The listing builds one solid part. Answer for the finished solid, in the listing's coordinates (mm). Face numbers are marked on the shaded views. A direction names the side the tool comes from. Round coordinates to 2 decimals unless told otherwise and drop trailing zeros. Order: outer loops, then holes, each group sorted by start corner. A loop starts at its lowest first (then second) coordinate and runs counter-clockwise, first axis right, second up. Notation, with made-up numbers: (27, 66.25) - (80, 66.25) arc R13 ccw to (80, 81.25) - close; hole circle Ø5 at (25, -21.75). An arc over 180 degrees is marked (long way). Use CSV: the item, a comma, the result in double quotes. Start each with the question number.
Item 1: Find section B-B, the plane x = 32.5. Give the vertices of the cut face in (y, z).
Item 2: For the marked faces 1 and 2, determine the directions among +Z, -Z, +X, -X, +Y, -Y from which every point of the face is accessible in a straight line to the end or side of a thin tool.
Item 3: Straight lines are drawn through the part: line 1 along Z through (x, y) = (4, 6); line 2 along X through (y, z) = (39, 47.5); line 3 along Y through (x, z) = (4, 23). For each, find the intervals that lie inside material, in ascending order. Write a range as [from, to].
Item 4: Find section D-D, the plane z = -72. Give the vertices of the cut face in (x, y).
Item 5: Find section A-A, the plane y = 20. Give the vertices of the cut face in (x, z), plus the area to 3 significant figures.
Item 6: Flat-ended cylindrical pins translate along their axes: P1, Ø6, axis at x = 10, y = 13.5, coming from the -Z side; P2, Ø10, axis at y = 57.5, z = 31, coming from the +X side; P3, Ø5, axis at x = 3.5, z = 37.5, coming from the +Y side; P4, Ø1.4, axis at x = 2.5, z = -27.5, coming from the -Y side. Find the tip coordinate at first contact, or state that the pin passes through.
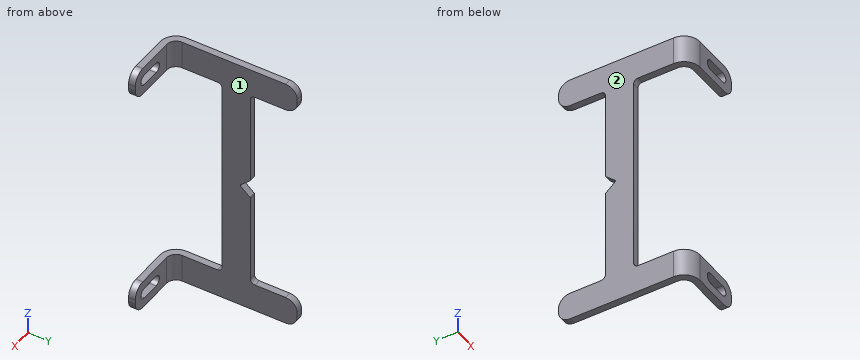
```python
from build123d import *

# Parameters (mm, degrees)
BASE_FLANGE1_DEPTH = 88.9
EXTRUDE2_REACH     = 132.358
EXTRUDE3_REACH     = 133.902
EXTRUDE4_DEPTH     = 134.35
FILLET1_R          = 7.9375
CUT_EXTRUDE1_REACH = 133.902
FILLET2_R          = 0.79375


# Sheet-metal steps are written as plain solids
with BuildPart() as part:
    # Sketch1 → Base-Flange1 (new, symmetric)
    with BuildSketch(Plane.XY):
        with BuildLine():
            Line((0, 88.9), (0, 10.90422))
            ThreePointArc((0, 10.90422), (3.193772094, 3.193772094), (10.90422, 0))
            Line((10.90422, 0), (44.45, 0))
            Line((44.45, 0), (44.45, 4.55422))
            Line((44.45, 4.55422), (10.90422, 4.55422))
            ThreePointArc((10.90422, 4.55422), (6.414091939, 6.414091939), (4.55422, 10.90422))
            Line((4.55422, 10.90422), (4.55422, 88.9))
            Line((4.55422, 88.9), (0, 88.9))
        make_face()
    extrude(amount=BASE_FLANGE1_DEPTH, both=True)

    # Sketch3 → Extrude2 (cut, up to next)
    with BuildSketch(Plane(origin=(0, 4.55422, 0), x_dir=(1, 0, 0), z_dir=(0, 1, 0)), mode=Mode.PRIVATE) as extrude2_sk1:
        with BuildLine():
            Line((34.925, -82.946875), (22.225, -82.946875))
            ThreePointArc((22.225, -82.946875), (18.653125, -79.375), (22.225, -75.803125))
            Line((22.225, -75.803125), (34.925, -75.803125))
            ThreePointArc((34.925, -75.803125), (38.496875, -79.375), (34.925, -82.946875))
        make_face()
    extrude2_tool1 = extrude(extrude2_sk1.sketch, amount=-EXTRUDE2_REACH, mode=Mode.PRIVATE) & part.part
    # Sketch3 → Extrude2 (cut, up to next)
    with BuildSketch(Plane(origin=(0, 4.55422, 0), x_dir=(1, 0, 0), z_dir=(0, 1, 0)), mode=Mode.PRIVATE) as extrude2_sk2:
        with BuildLine():
            Line((34.925, 75.803125), (22.225, 75.803125))
            ThreePointArc((22.225, 75.803125), (18.653125, 79.375), (22.225, 82.946875))
            Line((22.225, 82.946875), (34.925, 82.946875))
            ThreePointArc((34.925, 82.946875), (38.496875, 79.375), (34.925, 75.803125))
        make_face()
    extrude2_tool2 = extrude(extrude2_sk2.sketch, amount=-EXTRUDE2_REACH, mode=Mode.PRIVATE) & part.part
    add(extrude2_tool1.solids().sort_by_distance((28.575, 4.55422, 79.375))[0], mode=Mode.SUBTRACT)
    add(extrude2_tool2.solids().sort_by_distance((28.575, 4.55422, -79.375))[0], mode=Mode.SUBTRACT)

    # Sketch4 → Extrude3 (cut, up to next)
    with BuildSketch(Plane(origin=(4.55422, 0, 0), x_dir=(0, 0, -1), z_dir=(1, 0, 0)), mode=Mode.PRIVATE) as extrude3_sk1:
        with BuildLine():
            Line((-69.85, 88.9), (69.85, 88.9))
            Line((69.85, 88.9), (69.85, 60.325))
            ThreePointArc((69.85, 60.325), (68.92006403, 58.07993597), (66.675, 57.15))
            Line((66.675, 57.15), (-66.675, 57.15))
            ThreePointArc((-66.675, 57.15), (-68.92006403, 58.07993597), (-69.85, 60.325))
            Line((-69.85, 60.325), (-69.85, 88.9))
        make_face()
    extrude3_tool1 = extrude(extrude3_sk1.sketch, amount=-EXTRUDE3_REACH, mode=Mode.PRIVATE) & part.part
    add(extrude3_tool1.solids().sort_by_distance((4.55422, 73.039808, 0))[0], mode=Mode.SUBTRACT)

    # Sketch5 → Extrude4 (cut, through all)
    with BuildSketch(Plane.ZY):
        with BuildLine():
            Line((-66.675, 38.1), (66.675, 38.1))
            ThreePointArc((66.675, 38.1), (68.92006403, 37.17006403), (69.85, 34.925))
            Line((69.85, 34.925), (69.85, 0))
            Line((69.85, 0), (-69.85, 0))
            Line((-69.85, 0), (-69.85, 34.925))
            ThreePointArc((-69.85, 34.925), (-68.92006403, 37.17006403), (-66.675, 38.1))
        make_face()
    extrude(amount=-EXTRUDE4_DEPTH, mode=Mode.SUBTRACT)

    # Fillet1
    fillet1_edges = [part.edges().sort_by_distance(p)[0] for p in [
        (2.27711, 88.9, 88.9),
        (2.27711, 88.9, 69.85),
        (2.27711, 88.9, -69.85),
        (44.45, 2.27711, 88.9),
        (2.27711, 88.9, -88.9),
        (44.45, 2.27711, -88.9),
        (44.45, 2.27711, 69.85),
        (44.45, 2.27711, -69.85),
    ]]
    fillet(fillet1_edges, radius=FILLET1_R)

    # Sketch6 → Cut-Extrude1 (cut, up to next)
    with BuildSketch(Plane(origin=(4.55422, 0, 0), x_dir=(0, 0, -1), z_dir=(1, 0, 0)), mode=Mode.PRIVATE) as cut_extrude1_sk1:
        Polygon((-6.35, 57.15), (6.35, 57.15), (0, 50.00625), align=None)
    cut_extrude1_tool1 = extrude(cut_extrude1_sk1.sketch, amount=-CUT_EXTRUDE1_REACH, mode=Mode.PRIVATE) & part.part
    add(cut_extrude1_tool1.solids().sort_by_distance((4.55422, 54.76875, 0))[0], mode=Mode.SUBTRACT)

    # Fillet2
    fillet2_edges = [part.edges().sort_by_distance(p)[0] for p in [
        (2.27711, 50.00625, 0),
        (2.27711, 57.15, 6.35),
        (2.27711, 57.15, -6.35),
    ]]
    fillet(fillet2_edges, radius=FILLET2_R)


solid = part.part
```
Worked out:
1,outline,"(0, -88.9) - (4.55, -88.9) - (4.55, -82.95) - (0, -82.95) - close; (0, -75.8) - (4.55, -75.8) - (4.55, -69.85) - (0, -69.85) - close; (0, 69.85) - (4.55, 69.85) - (4.55, 75.8) - (0, 75.8) - close; (0, 82.95) - (4.55, 82.95) - (4.55, 88.9) - (0, 88.9) - close"
2,face 1,"+Z, -Z, +X, +Y"
2,face 2,"+Z, -Z, -X, +Y, -Y"
3,line 1,"z = [-88.9, -69.85], [69.85, 88.9]"
3,line 2,"x = [0, 4.55]"
3,line 3,"y = [38.1, 57.15]"
4,outline,"(0, 10.9) arc R10.9 ccw to (10.9, 0) - (41.94, 0) - (41.94, 4.55) - (10.9, 4.55) arc R6.35 cw to (4.55, 10.9) - (4.55, 86.39) - (0, 86.39) - close"
5,outline,"(0, -88.9) - (4.55, -88.9) - (4.55, -69.85) - (0, -69.85) - close; (0, 69.85) - (4.55, 69.85) - (4.55, 88.9) - (0, 88.9) - close"
5,area,"174 mm²"
6,P1,"passes through"
6,P2,"stops at x = 4.55"
6,P3,"stops at y = 57.15"
6,P4,"stops at y = 38.1"
